from build123d import *

# Parameters (mm, degrees)
F0_R      = 10
F1_DEPTH  = 320
F4_DEPTH  = 6
F6_R      = 10
F6_R_2    = 9.5
F7_DEPTH  = 1.35
F9_R      = 10
F9_R_2    = 9.5
F10_DEPTH = 1.35


with BuildPart() as f1:
    # F0 (on Front) → F1 (new body)
    with BuildSketch(Plane.XZ):
        Circle(F0_R)
    extrude(amount=F1_DEPTH)

    # F3 (on offset) → F4 (cut)
    with BuildSketch(Plane.XY.offset(12.5)):
        with BuildLine():
            Line((-3, -163.1), (-3, -230.9))
            Line((-3, -230.9), (3, -230.9))
            Line((3, -230.9), (3, -163.1))
            ThreePointArc((3, -163.1), (0, -166.1), (-3, -163.1))
        make_face()
        with BuildLine():
            ThreePointArc((3, -89.1), (0, -86.1), (-3, -89.1))
            Line((-3, -89.1), (3, -89.1))
        make_face()
        with BuildLine():
            Line((3, -230.9), (-3, -230.9))
            ThreePointArc((-3, -230.9), (0, -233.9), (3, -230.9))
        make_face()
        with BuildLine():
            Line((-3, -89.1), (-3, -156.9))
            ThreePointArc((-3, -156.9), (0, -153.9), (3, -156.9))
            Line((3, -156.9), (3, -89.1))
            Line((3, -89.1), (-3, -89.1))
        make_face()
        with BuildLine():
            ThreePointArc((3, -156.9), (0, -153.9), (-3, -156.9))
            ThreePointArc((-3, -156.9), (0, -159.9), (3, -156.9))
        make_face()
        with BuildLine():
            ThreePointArc((3, -163.1), (0, -160.1), (-3, -163.1))
            ThreePointArc((-3, -163.1), (0, -166.1), (3, -163.1))
        make_face()
    extrude(amount=-F4_DEPTH, mode=Mode.SUBTRACT)

    # F6 (on offset) → F7 (cut)
    with BuildSketch(Plane.XZ.offset(86)):
        Circle(F6_R)
        Circle(F6_R_2, mode=Mode.SUBTRACT)
    extrude(amount=-F7_DEPTH, mode=Mode.SUBTRACT)

    # F9 (on offset) → F10 (cut)
    with BuildSketch(Plane.XZ.offset(234)):
        Circle(F9_R)
        Circle(F9_R_2, mode=Mode.SUBTRACT)
    extrude(amount=F10_DEPTH, mode=Mode.SUBTRACT)


solid = f1.part
Could you check a few things on this model? Use its own coordinates, in mm. A direction names the side the tool comes from. Give positions to 0.01 mm unless a question says otherwise; leave off trailing zeros. Order: outer loops, then holes, each group sorted by start corner. A loop starts at its lowest first (then second) coordinate and runs counter-clockwise, first axis right, second up. Notation, with made-up numbers: (46, -17) - (97, -17) arc R22 cw to (97, 21) - close; hole circle Ø1 at (-35.75, -24). An arc over 180 degrees is marked (long way). One line per item, written item: value. Start each with the question number.
1. For P1, Ø3, axis at x = 0, y = -211.5, coming from the +Z side; P2, Ø4, axis at y = -163.5, z = -6, coming from the +X side; P3, Ø3, axis at y = -154, z = -4, coming from the +X side, each with a flat end and sliding along its axis, tell me the tip position at first contact or that it passes through.
2. Thinking about a two-plate mould opening in Y: for faces 1 (the face through (4.38, -85.33, -8.43)), 2 (the face through (0, -320, 0)), 3 (the face through (-2.17, -41.73, -9.76)), 4 (the face through (4.38, -234.67, -8.43)), which applies, +Y half, -Y half, draft (parallel to the pull), parting line (faces both ways), or undercut?
3. Imagine slicing it at C-C on z = -3.5. List the corners of the cut face in (x, y) for me, plus the area to 3 significant figures.
4. Imagine slicing it at B-B on y = -43.5. List the corners of the cut face in (x, z) for me, plus the area to 3 significant figures.
5. If I drill on probe 1 along Y at (x, z) = (-4.75, -8.75); probe 2 along Y at (x, z) = (2.75, 7); probe 3 along X at (y, z) = (-157, -0.75), over which ranges is the centre line in solid material (lowest first)?
6. Imagine slicing it at D-D on y = -184. List the corners of the cut face in (x, z) for me.
7. For faces 5 (the face through (0, -122, 6.5)), 6 (the face through (9, -235.35, -4)), 7 (the face through (-2.17, -158.96, -9.76)), which set-ups out of +Z, -Z, +X, -X, +Y, -Y let a thin tool reach every point of the face, with its end or its side?
8. Imagine slicing it at A-A on x = 0. List the corners of the cut face in (y, z) for me.
Values:
1. P1: z = 6.5
1. P2: x = 9.17
1. P3: x = 9.68
2. face 1: undercut
2. face 2: -Y half
2. face 3: draft
2. face 4: undercut
3. outline: (-9.37, -320) - (9.37, -320) - (9.37, -235.35) - (8.83, -235.35) - (8.83, -234) - (9.37, -234) - (9.37, -86) - (8.83, -86) - (8.83, -84.65) - (9.37, -84.65) - (9.37, 0) - (-9.37, 0) - (-9.37, -84.65) - (-8.83, -84.65) - (-8.83, -86) - (-9.37, -86) - (-9.37, -234) - (-8.83, -234) - (-8.83, -235.35) - (-9.37, -235.35) - close
3. area: 5,990 mm²
4. outline: circle Ø20 at (0, 0)
4. area: 314 mm²
5. probe 1: -320 to -235.35, -234 to -86, -84.65 to 0
5. probe 2: -320 to -232.1, -161.9 to -158.1, -87.9 to 0
5. probe 3: -9.97 to 9.97
6. outline: (-3, 6.5) - (-3, 9.54) arc R10 ccw (long way) to (3, 9.54) - (3, 6.5) - close
7. face 5: +Z
7. face 6: none
7. face 7: +Y, -Y
8. outline: (-320, -10) - (-235.35, -10) - (-235.35, -9.5) - (-234, -9.5) - (-234, -10) - (-86, -10) - (-86, -9.5) - (-84.65, -9.5) - (-84.65, -10) - (0, -10) - (0, 10) - (-84.65, 10) - (-84.65, 9.5) - (-86, 9.5) - (-86, 10) - (-86.1, 10) - (-86.1, 6.5) - (-159.9, 6.5) - (-159.9, 10) - (-160.1, 10) - (-160.1, 6.5) - (-233.9, 6.5) - (-233.9, 10) - (-234, 10) - (-234, 9.5) - (-235.35, 9.5) - (-235.35, 10) - (-320, 10) - close
